```python
from build123d import *

# Parameters (mm, degrees)
SKETCH1_R           = 1.75
BOSS_EXTRUDE1_DEPTH = 16.5
SKETCH2_W           = 3
SKETCH2_H           = 1
FILLET1_R           = 0.5


with BuildPart() as part:
    # Sketch1 → Boss-Extrude1 (new body)
    with BuildSketch(Plane(origin=(0, 0, 0), x_dir=(1, 0, 0), z_dir=(0, 1, 0))):
        with Locations(Location((0, 0, 0), (0, 0, 270))):
            Circle(SKETCH1_R)
    extrude(amount=BOSS_EXTRUDE1_DEPTH)

    # Sketch2 → Revolve1 (revolve)
    with BuildSketch(Plane.XY, mode=Mode.PRIVATE) as revolve1_sk:
        with Locations((-1.5, 17)):
            Rectangle(SKETCH2_W, SKETCH2_H)
        with Locations((-1.5, -0.5)):
            Rectangle(SKETCH2_W, SKETCH2_H)
    revolve(revolve1_sk.sketch.rotate(Axis((0, 0, 0), (0, 1, 0)), 270), axis=Axis((0, 0, 0), (0, 1, 0)))

    # Fillet1
    fillet1_edges = [part.edges().sort_by_distance(p)[0] for p in [
        (0, -1, 3),
        (0, 17.5, 3),
    ]]
    fillet(fillet1_edges, radius=FILLET1_R)


solid = part.part
```
Geometry: final body of the model. Coordinates: model frame, mm. A direction names the side the tool comes from. Round coordinates to 2 decimals unless told otherwise and drop trailing zeros. Order: outer loops, then holes, each group sorted by start corner. A loop starts at its lowest first (then second) coordinate and runs counter-clockwise, first axis right, second up. Notation, with made-up numbers: (-2.75, -35) -> (7.25, -35) arc R8 cw to (7.25, -23) -> close; hole circle Ø3 at (34.5, 80). An arc over 180 degrees is marked (long way). Use CSV: the item, a comma, the result in double quotes. Start each with the question number.
1) Section C-C (y = 2). Return the cut outline in (x, z), and give its area (3 significant figures).
2) Material intervals for line 1 along Y through (x, z) = (1.5, -1); line 2 along Y through (x, z) = (-2.8, -0.75); line 3 along Z through (x, y) = (1.2, 11.25), sorted ascending. Write a range as from..to.
3) Draft query along Y for faces 3 (the face through (-1.71, 8.13, -0.38)), 4 (the face through (-0.9, 16.75, -2.86)), 5 (the face through (2, 0, 0)), 6 (the face through (0, -1, 0)). Return one class per face: +Y half, -Y half, draft (parallel to the pull), parting line (faces both ways), or undercut.
4) First-contact query: pin 1 Ø1.5 at (x, y) = (0, 15.5) entering from -Z; pin 2 Ø1.5 at (x, y) = (-1.5, 15) entering from +Z; pin 3 Ø1.5 at (y, z) = (11, 1.5) entering from +X. Flat tips, straight axial feed; report the tip coordinate or a pass-through.
5) Section B-B (z = 0). Return the cut outline in (x, y), and give its area (3 significant figures).
6) Set-up query: faces 1 (the face through (2, 16.5, 0)), 2 (the face through (-0.9, -0.25, -2.86)). Return all of +Z, -Z, +X, -X, +Y, -Y with unobstructed straight access to the full face (end or side cutting, diameter ignored); none if empty.
7) Section A-A (x = 0). Return the cut outline in (y, z).
Returned:
1,outline,"circle Ø3.5 at (0, 0)"
1,area,"9.62 mm²"
2,line 1,"y = -1..0, 16.5..17.5"
2,line 2,"y = -0.8..0, 16.5..17.3"
2,line 3,"z = -1.27..1.27"
3,face 3,"undercut"
3,face 4,"draft"
3,face 5,"undercut"
3,face 6,"-Y half"
4,pin 1,"stops at z = -1.75"
4,pin 2,"stops at z = 1.58"
4,pin 3,"stops at x = 1.58"
5,outline,"(-3, -0.5) arc R0.5 ccw to (-2.5, -1) -> (2.5, -1) arc R0.5 ccw to (3, -0.5) -> (3, 0) -> (1.75, 0) -> (1.75, 16.5) -> (3, 16.5) -> (3, 17) arc R0.5 ccw to (2.5, 17.5) -> (-2.5, 17.5) arc R0.5 ccw to (-3, 17) -> (-3, 16.5) -> (-1.75, 16.5) -> (-1.75, 0) -> (-3, 0) -> close"
5,area,"69.5 mm²"
6,face 1,"none"
6,face 2,"+Y, -Y"
7,outline,"(-1, -2.5) arc R0.5 ccw to (-0.5, -3) -> (0, -3) -> (0, -1.75) -> (16.5, -1.75) -> (16.5, -3) -> (17, -3) arc R0.5 ccw to (17.5, -2.5) -> (17.5, 2.5) arc R0.5 ccw to (17, 3) -> (16.5, 3) -> (16.5, 1.75) -> (0, 1.75) -> (0, 3) -> (-0.5, 3) arc R0.5 ccw to (-1, 2.5) -> close"
